from build123d import *

# Parameters (mm, degrees)
BOSS_EXTRUDE1_DEPTH = 3
CUT_EXTRUDE1_DEPTH  = 3


with BuildPart() as part:
    # Sketch1 → Boss-Extrude1 (new body)
    with BuildSketch(Plane(origin=(766.479324321, -257.616944778, 0), x_dir=(0.26047542598858736, 0.9654804775116191, 0), z_dir=(0, 0, 1))):
        Polygon((33.772102577, 853.041764539), (33.772102577, 816.600953816), (49.075102345, 807.123707481), (118.453517154, 919.149693533), (76.300457153, 921.712703038), align=None)
    extrude(amount=BOSS_EXTRUDE1_DEPTH)

    # Sketch2 → Cut-Extrude1 (cut)
    with BuildSketch(Plane(origin=(0, 0, 3), x_dir=(0.26047542598858736, 0.965480477511619, 0), z_dir=(0, 0, 1))):
        with BuildLine():
            Line((20.841316823, 91.584158174), (50.525265903, 89.779301217))
            ThreePointArc((50.525265903, 89.779301217), (53.172383437, 92.122966884), (50.82871777, 94.770084418))
            Line((50.82871777, 94.770084418), (21.144768691, 96.574941376))
            ThreePointArc((21.144768691, 96.574941376), (18.497651156, 94.231275709), (20.841316823, 91.584158174))
        make_face()
        with BuildLine():
            Line((14.861969696, 81.929249515), (44.545918775, 80.124392558))
            ThreePointArc((44.545918775, 80.124392558), (47.19303631, 82.468058225), (44.849370643, 85.115175759))
            Line((44.849370643, 85.115175759), (15.165421563, 86.920032717))
            ThreePointArc((15.165421563, 86.920032717), (12.518304029, 84.57636705), (14.861969696, 81.929249515))
        make_face()
        with BuildLine():
            Line((27.124115818, 106.229850035), (56.808064898, 104.424993077))
            ThreePointArc((56.808064898, 104.424993077), (59.151730565, 101.777875543), (56.50461303, 99.434209876))
            Line((56.50461303, 99.434209876), (26.82066395, 101.239066833))
            ThreePointArc((26.82066395, 101.239066833), (24.476998283, 103.886184368), (27.124115818, 106.229850035))
        make_face()
        with BuildLine():
            Line((8.882622568, 72.274340856), (38.566571648, 70.469483899))
            ThreePointArc((38.566571648, 70.469483899), (41.213689182, 72.813149566), (38.870023515, 75.4602671))
            Line((38.870023515, 75.4602671), (9.186074436, 77.265124058))
            ThreePointArc((9.186074436, 77.265124058), (6.538956901, 74.921458391), (8.882622568, 72.274340856))
        make_face()
        with BuildLine():
            Line((2.903275441, 62.619432197), (32.58722452, 60.814575239))
            ThreePointArc((32.58722452, 60.814575239), (35.234342055, 63.158240906), (32.890676388, 65.805358441))
            Line((32.890676388, 65.805358441), (3.206727308, 67.610215399))
            ThreePointArc((3.206727308, 67.610215399), (0.559609774, 65.266549732), (2.903275441, 62.619432197))
        make_face()
        with BuildLine():
            Line((-3.076071687, 52.964523538), (26.607877393, 51.15966658))
            ThreePointArc((26.607877393, 51.15966658), (29.254994927, 53.503332247), (26.911329261, 56.150449782))
            Line((26.911329261, 56.150449782), (-2.772619819, 57.95530674))
            ThreePointArc((-2.772619819, 57.95530674), (-5.419737354, 55.611641073), (-3.076071687, 52.964523538))
        make_face()
        with BuildLine():
            Line((-9.055418814, 43.309614879), (20.628530266, 41.504757921))
            ThreePointArc((20.628530266, 41.504757921), (23.2756478, 43.848423588), (20.931982133, 46.495541123))
            Line((20.931982133, 46.495541123), (-8.751966947, 48.30039808))
            ThreePointArc((-8.751966947, 48.30039808), (-11.399084481, 45.956732414), (-9.055418814, 43.309614879))
        make_face()
        with BuildLine():
            Line((-9.651273834, 38.336610507), (14.952635006, 36.840632464))
            ThreePointArc((14.952635006, 36.840632464), (17.296300673, 34.193514929), (14.649183138, 31.849849262))
            Line((14.649183138, 31.849849262), (-9.954725702, 33.345827305))
            ThreePointArc((-9.954725702, 33.345827305), (-12.298391369, 35.99294484), (-9.651273834, 38.336610507))
        make_face()
        with BuildLine():
            Line((-9.651273834, 28.318142867), (8.973287878, 27.185723805))
            ThreePointArc((8.973287878, 27.185723805), (11.316953545, 24.53860627), (8.669836011, 22.194940603))
            Line((8.669836011, 22.194940603), (-9.954725702, 23.327359666))
            ThreePointArc((-9.954725702, 23.327359666), (-12.298391369, 25.9744772), (-9.651273834, 28.318142867))
        make_face()
        with BuildLine():
            Line((-9.651273834, 18.299675228), (2.993940751, 17.530815146))
            ThreePointArc((2.993940751, 17.530815146), (5.337606418, 14.883697611), (2.690488883, 12.540031944))
            Line((2.690488883, 12.540031944), (-9.954725702, 13.308892026))
            ThreePointArc((-9.954725702, 13.308892026), (-12.298391369, 15.956009561), (-9.651273834, 18.299675228))
        make_face()
    extrude(amount=-CUT_EXTRUDE1_DEPTH, mode=Mode.SUBTRACT)


solid = part.part
Source: CAD feature listing. Evaluate the final solid. Frame: model axes, mm. Round coordinates to 2 decimals unless told otherwise and drop trailing zeros. Loops run counter-clockwise (first coordinate to the right, second up) from the corner with the lowest first, then second, coordinate; pieces in that order, holes last.
Q1. Section B-B, the plane z = 1.1. State how many separate pieces and enclosed holes the cut face has, plus the area to 3 significant figures.
Q2. Mould query, pull axis X, two halves, no side actions, for faces 1 (the face through (-55.156, 9.271, 1.521)), 2 (the face through (-76.317, 27.072, 1.479)). Classes: pulls with the +X half, pulls with the -X half, needs draft (parallel to the pull), parting line crosses it, or undercut.
Q3. Section A-A, the plane y = 62.5. Return loops of the section in (x, z), plus the area to 3 significant figures.
Q4. First-contact query: P1, Ø2, axis at x = -82.5, y = 61, coming from the +Z side; P2, Ø1.5, axis at y = 80, z = 0.5, coming from the -X side; P3, Ø1, axis at x = -89.5, y = 68, coming from the -Z side. Flat tips, straight axial feed; report the tip coordinate or a pass-through.
Q5. Ray query, line 1 (X direction, y = 35.5, z = 2.1); line 2 (X direction, y = 62, z = 2.25); line 3 (X direction, y = 46.5, z = 2.5). Return the intervals inside material, ascending.
Q6. Section C-C, the plane y = 87.5. Return loops of the section in (x, z).
Solutions:
1. separate pieces: 1
1. enclosed holes: 10
1. area: 2,710 mm2
2. face 1: undercut
2. face 2: pulls with the -X half
3. outline: (-101.4, 0) - (-92.59, 0) - (-92.59, 3) - (-101.4, 3) - close; (-87.32, 0) - (-82.04, 0) - (-82.04, 3) - (-87.32, 3) - close; (-76.77, 0) - (-71.49, 0) - (-71.49, 3) - (-76.77, 3) - close; (-66.22, 0) - (-58.55, 0) - (-58.55, 3) - (-66.22, 3) - close
3. area: 81.1 mm2
4. P1: stops at z = 3
4. P2: stops at x = -95.77
4. P3: passes through
5. line 1: x = -84.21 to -79.9, -75.3 to -70.02, -64.74 to -59.47, -54.19 to -48.92, -43.64 to -33.26
5. line 2: x = -101.57 to -92.76, -87.49 to -82.21, -76.94 to -71.66, -66.39 to -58.08
5. line 3: x = -94.52 to -87.42, -82.15 to -76.87, -71.6 to -66.32, -61.05 to -55.77, -50.5 to -43.56
6. outline: (-93, 0) - (-81.97, 0) - (-81.97, 3) - (-93, 3) - close
